Autodesk Inventor part; units mm, degrees
ref_plane "YZ Plane" through (0, 0, 0) normal (1, 0, 0) x (0, 1, 0)
ref_plane "XZ Plane" through (0, 0, 0) normal (0, 1, 0) x (-1, 0, 0)
ref_plane "XY Plane" through (0, 0, 0) normal (0, 0, 1) x (1, 0, 0)
sketch "スケッチ1" plane through (0, 0, 0) normal (0, 1, 0) x (-1, 0, 0)
  line L0 (0, 0) -> (32, 0)
  line L1 (32, 0) -> (32, -43)
  line L2 (32, -43) -> (0, -43)
  line L3 (0, -43) -> (0, 0)
  dimension "d0" = 32
  dimension "d1" = 43
extrude "押し出し1" add sketch "スケッチ1" along normal blind 32.5
sketch "スケッチ2" plane through (0, 0, 0) normal (0, -1, 0) x (1, 0, 0)
  line L0 (-32, -43) -> (-32, 0) construction
  line L1 (-32, -21.5) -> (0, -21.5) construction
  line L2 (0, 0) -> (0, -43) construction
  line L3 (-16, -21.5) -> (-16, -12) construction
  line L4 (-32, 0) -> (-32, -43)
  arc A0 (-26.583, 0) -> (-32, -12) centre (-16, -12) ccw
  arc A1 (0, -12) -> (-5.417, 0) centre (-16, -12) ccw
  line L5 (-32, -12) -> (-32, 0)
  line L6 (0, 0) -> (-32, 0)
  line L7 (-5.417, 0) -> (0, 0)
  line L8 (0, 0) -> (0, -12)
  line L9 (-32, 0) -> (-26.583, 0)
  dimension "d4" = 9.5
extrude "押し出し2" cut sketch "スケッチ2" against normal blind 32.5
sketch "スケッチ3" plane through (0, 0, 0) normal (0, -1, 0) x (1, 0, 0)
  line L0 (-32, -21.5) -> (0, -21.5) construction
  line L1 (0, -21.5) -> (0, -43) construction
  line L2 (-5.417, 0) -> (-26.583, 0) construction
  line L3 (-16, 0) -> (-16, -43) construction
  line L4 (-32, -43) -> (0, -43) construction
  line L5 (-16, -21.5) -> (-16, -13) construction
  line L6 (-16, -21.5) -> (-29.5, -21.5) construction
  circle A0 centre (-29.5, -13) radius 1
  line L7 (-16, -21.5) -> (-2.5, -21.5) construction
  circle A1 centre (-2.5, -13) radius 1
  line L8 (-16, -21.5) -> (-16, -40) construction
  circle A2 centre (-29.5, -40) radius 1
  circle A3 centre (-2.5, -40) radius 1
  point P0 (0, 0)
  dimension "d8" = 8.5
  dimension "d9" = 13.5
  dimension "d10" = 2
  dimension "d11" = 13.5
  dimension "d12" = 2
  dimension "d13" = 18.5
  dimension "d14" = 2
  dimension "d15" = 2
extrude "押し出し3" cut sketch "スケッチ3" against normal blind 32.5
sketch "スケッチ4" plane through (0, 32.5, 0) normal (0, 1, 0) x (1, 0, 0)
  line L0 (-5.417, 0) -> (-26.583, 0) construction
  line L1 (-32, 21.5) -> (0, 21.5) construction
  line L2 (0, 21.5) -> (0, 43) construction
  line L3 (-16, 0) -> (-16, 43) construction
  line L4 (-32, 43) -> (0, 43) construction
  line L5 (-16, 21.5) -> (-16, 13) construction
  line L6 (-16, 21.5) -> (-29.5, 21.5) construction
  circle A0 centre (-29.5, 13) radius 1
  line L7 (-16, 21.5) -> (-2.5, 21.5) construction
  circle A1 centre (-2.5, 13) radius 1
  line L8 (-16, 21.5) -> (-16, 40) construction
  circle A2 centre (-29.5, 40) radius 1
  circle A3 centre (-2.5, 40) radius 1
  line L9 (-29.5, 21.5) -> (-29.5, 22) construction
  line L10 (-2.5, 21.5) -> (-2.5, 35) construction
  line L11 (-16, 21.5) -> (-16, 4.5) construction
  line L12 (-16, 4.5) -> (-5, 4.5) construction
  line L13 (-16, 4.5) -> (-27, 4.5) construction
  circle A4 centre (-2.5, 35) radius 1
  circle A5 centre (-29.5, 22) radius 1
  circle A6 centre (-27, 4.5) radius 1
  circle A7 centre (-5, 4.5) radius 1
  line L14 (0, 43) -> (-32, 43)
  line L15 (0, 43) -> (-32, 43)
  line L16 (-32, 43) -> (-32, 12)
  line L17 (-32, 43) -> (-32, 12)
  line L18 (0, 12) -> (0, 43)
  line L19 (0, 43) -> (0, 12)
  line L20 (-26.583, 0) -> (-5.417, 0)
  line L21 (-5.417, 0) -> (-26.583, 0)
  arc A8 (-32, 12) -> (-26.583, 0) centre (-16, 12) ccw
  arc A9 (-5.417, 0) -> (0, 12) centre (-16, 12) ccw
  arc A10 (-5.417, 0) -> (0, 12) centre (-16, 12) ccw
  circle A11 centre (-29.5, 40) radius 1 construction
  line L22 (-2.5, 40) -> (-29.5, 40) construction
  point P0 (0, 0)
  point P1 (0, 0)
  dimension "d26" = 0.5
  dimension "d27" = 13.5
  dimension "d28" = 17
  dimension "d29" = 11
  dimension "d30" = 11
  dimension "d31" = 2
  dimension "d32" = 2
  dimension "d33" = 2
  dimension "d34" = 2
extrude "押し出し4" cut sketch "スケッチ4" against normal blind 30 contours A4 | A5 | A6 | A7
sketch "スケッチ5" plane through (0, 0, 0) normal (0, -1, 0) x (1, 0, 0)
  line L0 (-32, -21.5) -> (0, -21.5) construction
  line L1 (0, -21.5) -> (0, -43) construction
  line L2 (-5.417, 0) -> (-26.583, 0) construction
  line L3 (-16, 0) -> (-16, -43) construction
  line L4 (-32, -43) -> (0, -43) construction
  line L5 (-16, -21.5) -> (-16, -12) construction
  line L6 (-16, -21.5) -> (-29.5, -21.5) construction
  circle A0 centre (-29.5, -13) radius 1
  line L7 (-16, -21.5) -> (-2.5, -21.5) construction
  circle A1 centre (-2.5, -13) radius 1
  line L8 (-16, -21.5) -> (-16, -40) construction
  circle A2 centre (-29.5, -40) radius 1
  circle A3 centre (-2.5, -40) radius 1
  circle A4 centre (-16, -12) radius 3
  point P0 (0, 0)
  point P1 (0, 0)
  dimension "d37" = 9.5
  dimension "d38" = 13.5
  dimension "d39" = 2
  dimension "d40" = 13.5
  dimension "d41" = 2
  dimension "d42" = 18.5
  dimension "d43" = 2
  dimension "d44" = 2
  dimension "d45" = 6
extrude "押し出し5" add sketch "スケッチ5" along normal blind 3 contours A4
sketch "スケッチ6" plane through (-16, -3, -12) normal (0, -1, 0) x (1, 0, 0)
  circle A0 centre (0, 0) radius 1.3
  point P0 (16, 12)
  dimension "d48" = 2.6
extrude "押し出し6" cut sketch "スケッチ6" against normal blind 7
sketch "スケッチ7" plane through (0, 32.5, 0) normal (0, 1, 0) x (1, 0, 0)
  line L0 (-5.417, 0) -> (-26.583, 0) construction
  line L1 (-16, 21.5) -> (-29.5, 21.5) construction
  line L2 (-16, 21.5) -> (-16, 13) construction
  line L3 (-16, 21.5) -> (-2.5, 21.5) construction
  line L4 (-32, 21.5) -> (0, 21.5) construction
  line L5 (-32, 43) -> (0, 43) construction
  line L6 (-16, 21.5) -> (-16, 40) construction
  line L7 (0, 21.5) -> (0, 43) construction
  line L8 (-16, 0) -> (-16, 43) construction
  line L9 (-29.5, 21.5) -> (-29.5, 22) construction
  line L10 (-16, 21.5) -> (-16, 12) construction
  line L11 (-16, 12) -> (-5, 12) construction
  line L12 (-16, 12) -> (-27, 12) construction
  circle A0 centre (-16, 12) radius 1.3
  circle A1 centre (-16, 12) radius 4.25
  point P0 (0, 0)
  point P1 (0, 0)
  point P2 (0, 0)
  dimension "d53" = 9.5
  dimension "d60" = 8.5
extrude "押し出し7" cut sketch "スケッチ7" against normal blind 0.5 contours A0 | A1
sketch "スケッチ8" plane through (-16, 32, -12) normal (0, 1, 0) x (1, 0, 0)
  circle A0 centre (0, 0) radius 2.7
  point P0 (16, -12)
  dimension "d63" = 5.4
extrude "押し出し8" add sketch "スケッチ8" along normal blind 0.5
sketch "スケッチ9" plane through (-16, 32.5, -12) normal (0, 1, 0) x (1, 0, 0)
  circle A0 centre (0, 0) radius 1.3
  point P0 (16, -12)
  dimension "d66" = 2.6
extrude "押し出し9" cut sketch "スケッチ9" against normal blind 10
sketch "スケッチ10" plane through (0, 0, -43) normal (1, 0, 0) x (0, 0, -1)
  line L0 (0, 0) -> (0, 32.5) construction
  line L1 (0, 0) -> (-31, 0) construction
  line L2 (-21.5, 27.5) -> (-27.2, 27.5)
  line L3 (-27.2, 27.5) -> (-27.2, 24.6)
  line L4 (-27.2, 24.6) -> (-18.5, 24.6)
  line L5 (-18.5, 24.6) -> (-18.5, 25.6)
  line L6 (-18.5, 25.6) -> (-19.5, 25.6)
  line L7 (-19.5, 25.6) -> (-19.5, 27.5)
  line L8 (-19.5, 27.5) -> (-21.5, 27.5)
  line L9 (-27.2, 24.6) -> (-27.2, 22.1)
  line L10 (-27.2, 22.1) -> (-18.5, 22.1)
  line L11 (-18.5, 22.1) -> (-18.5, 23.1)
  line L12 (-18.5, 23.1) -> (-19.5, 23.1)
  line L13 (-19.5, 23.1) -> (-19.5, 24.6)
  line L14 (0, 32.5) -> (-21.5, 32.5) construction
  line L15 (-31, 32.5) -> (0, 32.5) construction
  line L16 (-21.5, 32.5) -> (-21.5, 27.5) construction
  point P0 (-43, 0)
  dimension "d72" = 2.9
  dimension "d73" = 5.7
  dimension "d74" = 8.7
  dimension "d75" = 1
  dimension "d76" = 1
  dimension "d79" = 2.5
  dimension "d80" = 1
  dimension "d81" = 1
  dimension "d85" = 21.5
  dimension "d86" = 5
extrude "押し出し11" cut sketch "スケッチ10" against normal blind 10
properties part number "Servo"
Could you check a few things on this model? Use its own coordinates, in mm. A direction names the side the tool comes from. Give positions to 0.01 mm unless a question says otherwise; leave off trailing zeros. Loops run counter-clockwise (first coordinate to the right, second up) from the corner with the lowest first, then second, coordinate; pieces in that order, holes last. Notation, with made-up numbers: (21.5, -35.5) - (42.5, -35.5) arc R31 cw to (42.5, -6.5) - close; hole circle Ø6 at (57, 12). An arc over 180 degrees is marked (long way). Answer in a Markdown table with one row per item. Add a question column.
Q1. If we section it at C-C (x = -16): List the corners of the cut face in (y, z) for me.
Q2. For pin 1 (1 mm diameter, centred on x = -5.5, z = -14, fed in from -Y); pin 2 (1.2 mm diameter, centred on x = -2.5, z = -35, fed in from +Y); pin 3 (1.6 mm diameter, centred on x = -2.5, z = -40, fed in from +Y), each with a flat end and sliding along its axis, tell me the tip position at first contact or that it passes through.
Q3. We'd pull the mould along Y, two halves only. Please class faces 1 (the face through (-30.544, 16.022, -5.331)), 2 (the face through (-16, 4, -12)), 3 (the face through (-5, 25, -15.8)), 4 (the face through (-16, 22.5, -12)): +Y half, -Y half, draft (parallel to the pull), parting line (faces both ways), or undercut.
Q4. If we section it at A-A (z = -40): List the corners of the cut face in (x, y) for me.
Q5. If we section it at B-B (y = 19): State how many separate pieces and enclosed holes the cut face has, plus the area to 3 significant figures.
Q6. Which directions (+Z, -Z, +X, -X, +Y, -Y) give clear straight access to the entire face, cutting with the end or side of a thin tool? Please do faces 5 (the face through (-27, 2.5, -5)), 6 (the face through (-5, 24, -23.5)), 7 (the face through (-16, 16, -43)), 8 (the face through (-19, -1, -12)).
Q7. If we section it at D-D (x = -2.5): List the corners of the cut face in (y, z) for me.
Q8. Please list where these lines run through material, in increasing order: L1, parallel to Z at x = -16, y = 32.25; L2, parallel to X at y = 18, z = -4; L3, parallel to Z at x = -16, y = 28.5. Write a range as from..to.
The answers:
| question | item | result |
|---|---|---|
| 1 | outline | (-3, -15) - (0, -15) - (0, -43) - (32.5, -43) - (32.5, -16.25) - (32, -16.25) - (32, -14.7) - (32.5, -14.7) - (32.5, -13.3) - (22.5, -13.3) - (22.5, -10.7) - (32.5, -10.7) - (32.5, -9.3) - (32, -9.3) - (32, -7.75) - (32.5, -7.75) - (32.5, 0) - (0, 0) - (0, -9) - (-3, -9) - (-3, -10.7) - (4, -10.7) - (4, -13.3) - (-3, -13.3) - close |
| 2 | pin 1 | stops at y = 0 |
| 2 | pin 2 | stops at y = 2.5 |
| 2 | pin 3 | passes through |
| 3 | face 1 | draft |
| 3 | face 2 | -Y half |
| 3 | face 3 | undercut |
| 3 | face 4 | +Y half |
| 4 | outline | (-32, 0) - (-30.5, 0) - (-30.5, 32.5) - (-32, 32.5) - close; (-28.5, 0) - (-3.5, 0) - (-3.5, 32.5) - (-28.5, 32.5) - close; (-1.5, 0) - (0, 0) - (0, 32.5) - (-1.5, 32.5) - close |
| 5 | separate pieces | 1 |
| 5 | enclosed holes | 8 |
| 5 | area | 1,310 mm^2 |
| 6 | face 5 | +Y |
| 6 | face 6 | +X |
| 6 | face 7 | -Z, +X, -X, +Y, -Y |
| 6 | face 8 | -Y |
| 7 | outline | (0, -43) - (32.5, -43) - (32.5, -41) - (0, -41) - close; (0, -39) - (32.5, -39) - (32.5, -36) - (2.5, -36) - (2.5, -34) - (32.5, -34) - (32.5, -14) - (0, -14) - close; (0, -12) - (32.5, -12) - (32.5, -3.41) - (0, -3.41) - close; hole (22.1, -24.5) - (23.1, -24.5) - (23.1, -23.5) - (24.6, -23.5) - (24.6, -24.5) - (25.6, -24.5) - (25.6, -23.5) - (27.5, -23.5) - (27.5, -15.8) - (22.1, -15.8) - close |
| 8 | L1 | z = -43..-16.25, -14.7..-13.3, -10.7..-9.3, -7.75..0 |
| 8 | L2 | x = -29.86..-27.87, -26.13..-5.87, -4.13..-2.14 |
| 8 | L3 | z = -43..-13.3, -10.7..0 |
